Could you check a few things on this model? Use its own coordinates, in mm. A direction names the side the tool comes from. Coordinates: 2 decimals unless noted, no trailing zeros. Loops run counter-clockwise (first coordinate to the right, second up) from the corner with the lowest first, then second, coordinate; pieces in that order, holes last. Notation, with made-up numbers: M 13.25,13.25 L 52.25,13.25 A25 ccw 52.25,34.25 Z; hole C 75.5,31 d4. An arc over 180 degrees is marked long. Use one line per item in the form item = value. Start each with the question number.
```python
from build123d import *

# Parameters (mm, degrees)
SKETCH1_R           = 2.5
SKETCH1_R_2         = 2.1
SKETCH1_R_3         = 10.5
BOSS_EXTRUDE1_DEPTH = 2


with BuildPart() as part:
    # Sketch1 → Boss-Extrude1 (new body)
    with BuildSketch(Plane(origin=(0, 0, 0), x_dir=(1, 0, 0), z_dir=(0, 1, 0))):
        with BuildLine():
            Line((-35.525840533, 12), (-33.525840533, 12))
            ThreePointArc((-33.525840533, 12), (-33.133608263, 12.038838649), (-32.756609764, 12.153846154))
            ThreePointArc((-32.756609764, 12.153846154), (-28.525840533, 13), (-24.295071303, 12.153846154))
            ThreePointArc((-24.295071303, 12.153846154), (-23.918072804, 12.038838649), (-23.525840533, 12))
            Line((-23.525840533, 12), (-22.525840533, 12))
            ThreePointArc((-22.525840533, 12), (-18.990306627, 10.535533906), (-17.525840533, 7))
            Line((-17.525840533, 7), (-17.525840533, -4))
            ThreePointArc((-17.525840533, -4), (-18.990306627, -7.535533906), (-22.525840533, -9))
            Line((-22.525840533, -9), (-35.525840533, -9))
            ThreePointArc((-35.525840533, -9), (-36.940054096, -9.585786438), (-37.525840533, -11))
            Line((-37.525840533, -11), (-37.525840533, -34))
            ThreePointArc((-37.525840533, -34), (-36.940054096, -35.414213562), (-35.525840533, -36))
            Line((-35.525840533, -36), (-17.525840533, -36))
            ThreePointArc((-17.525840533, -36), (-13.990306627, -34.535533906), (-12.525840533, -31))
            Line((-12.525840533, -31), (-12.525840533, -21.5))
            ThreePointArc((-12.525840533, -21.5), (-11.061374439, -17.964466094), (-7.525840533, -16.5))
            Line((-7.525840533, -16.5), (11.525840533, -16.5))
            ThreePointArc((11.525840533, -16.5), (15.061374439, -15.035533906), (16.525840533, -11.5))
            Line((16.525840533, -11.5), (16.525840533, 15))
            ThreePointArc((16.525840533, 15), (15.061374439, 18.535533906), (11.525840533, 20))
            Line((11.525840533, 20), (-35.525840533, 20))
            ThreePointArc((-35.525840533, 20), (-36.940054096, 19.414213562), (-37.525840533, 18))
            Line((-37.525840533, 18), (-37.525840533, 14))
            ThreePointArc((-37.525840533, 14), (-36.940054096, 12.585786438), (-35.525840533, 12))
        make_face()
        with Locations((-11.525840533, 11.525840533)):
            Circle(SKETCH1_R, mode=Mode.SUBTRACT)
        with Locations((11.525840533, 11.525840533)):
            Circle(SKETCH1_R, mode=Mode.SUBTRACT)
        with Locations((11.525840533, -11.525840533)):
            Circle(SKETCH1_R, mode=Mode.SUBTRACT)
        with Locations((-11.525840533, -11.525840533)):
            Circle(SKETCH1_R, mode=Mode.SUBTRACT)
        with Locations((-33.525840533, 16)):
            Circle(SKETCH1_R_2, mode=Mode.SUBTRACT)
        with Locations((-23.525840533, 16)):
            Circle(SKETCH1_R_2, mode=Mode.SUBTRACT)
        with Locations((-33.525840533, -32)):
            Circle(SKETCH1_R_2, mode=Mode.SUBTRACT)
        with Locations((-23.525840533, -32)):
            Circle(SKETCH1_R_2, mode=Mode.SUBTRACT)
        with Locations((-33.525840533, -13)):
            Circle(SKETCH1_R_2, mode=Mode.SUBTRACT)
        with Locations((-23.525840533, -13)):
            Circle(SKETCH1_R_2, mode=Mode.SUBTRACT)
        Circle(SKETCH1_R_3, mode=Mode.SUBTRACT)
    extrude(amount=BOSS_EXTRUDE1_DEPTH)


solid = part.part
```
Item 1: Thinking about a two-plate mould opening in X: for faces 6 (the cylindrical face through (10, 1, -3.2)), 7 (the flat face through (-12, 1, -20)), 8 (the cylindrical face through (-36.924, 0.986, -19.43)), which applies, pulls with the +X half, pulls with the -X half, needs draft (parallel to the pull), parting line crosses it, or undercut?
Item 2: I want a section at D-D (z = -16). Write out the boundary of the cut face in (x, y).
Item 3: For faces 1 (the flat face through (-29, 1, 9)), 2 (the cylindrical face through (-36.956, 0.986, 35.399)), 3 (the cylindrical face through (-28.6, 1, -13)), 4 (the flat face through (-37.526, 1, 22)), 5 (the flat face through (2, 1, 16.5)), which set-ups out of +Z, -Z, +X, -X, +Y, -Y let a thin tool reach every point of the face, with its end or its side?
Item 4: Please list where these lines run through material, in increasing order: line 1 along X through (y, z) = (1.3, 12); line 2 along X through (y, z) = (1.3, 32); line 3 along Z through (x, y) = (-12, 0.45).
Item 5: I want a section at C-C (z = 32). Write out the boundary of the cut face in (x, y), plus the area to 3 significant figures.
Item 6: I want a section at A-A (z = 0). Write out the boundary of the cut face in (x, y).
Item 7: I want a section at B-B (x = 0). Write out the boundary of the cut face in (y, z).
Item 8: I'm going to push flat-ended pins straight in: P1, Ø1, axis at y = 1, z = -2.5, coming from the -X side; P2, Ø4, axis at x = -33.53, z = -16, coming from the +Y side; P3, Ø1, axis at y = 0, z = 9.5, coming from the -X side. Where does each tip first touch, or does it pass through?
Worked answers:
q1.face_6 = undercut
q1.face_7 = needs draft
q1.face_8 = pulls with the -X half
q2.outline = M -37.53,0 L -35.63,0 L -35.63,2 L -37.53,2 Z; M -31.43,0 L -25.63,0 L -25.63,2 L -31.43,2 Z; M -21.43,0 L 16.42,0 L 16.42,2 L -21.43,2 Z
q3.face_1 = -X, +Y, -Y
q3.face_2 = +Z, -X, +Y, -Y
q3.face_3 = +Y, -Y
q3.face_4 = +Z, -Z, -X, +Y, -Y
q3.face_5 = +Z, +X, +Y, -Y
q4.line_1 = -37.53 to -35.37, -31.68 to -25.37, -21.68 to -13.98, -9.07 to 9.07, 13.98 to 16.5
q4.line_2 = -37.53 to -35.63, -31.43 to -25.63, -21.43 to -12.63
q4.line_3 = -20 to -13.98, -9.07 to 9.07, 13.98 to 19.27
q5.outline = M -37.53,0 L -35.63,0 L -35.63,2 L -37.53,2 Z; M -31.43,0 L -25.63,0 L -25.63,2 L -31.43,2 Z; M -21.43,0 L -12.63,0 L -12.63,2 L -21.43,2 Z
q5.area = 33.0 mm²
q6.outline = M -17.53,0 L -10.5,0 L -10.5,2 L -17.53,2 Z; M 10.5,0 L 16.53,0 L 16.53,2 L 10.5,2 Z
q7.outline = M 0,-20 L 2,-20 L 2,-10.5 L 0,-10.5 Z; M 0,10.5 L 2,10.5 L 2,16.5 L 0,16.5 Z
q8.P1 = -17.53
q8.P2 = through
q8.P3 = -37.26
